```python
from build123d import *

# Parameters (mm, degrees)
EXTRUDE_START            = 27.5
EXTRUDE_1_DEPTH          = 55
SKETCH_4_R               = 10
CUT_EXTRUDE_1_DEPTH      = 55.60082417
CUT_EXTRUDE_2_DEPTH      = 55.60082417
CUT_EXTRUDE_2_DEPTH_BACK = 55.60082417
SKETCH_6_R               = 3.5
CUT_EXTRUDE_3_DEPTH      = 54.937463789
FILLET_1_R               = 2
FILLET_2_R               = 2.8


with BuildPart() as part:
    # 草图3 → 凸台-拉伸1 (new body)
    with BuildSketch(Plane(origin=(0, 0, 0), x_dir=(0, 0, -1), z_dir=(1, 0, 0)).offset(EXTRUDE_START)):
        with BuildLine():
            Line((-28, 0), (-5, 0))
            ThreePointArc((-5, 0), (-1.464466094, 1.464466094), (0, 5))
            Line((0, 5), (0, 40))
            Line((0, 40), (-3, 40))
            Line((-3, 40), (-3, 5))
            ThreePointArc((-3, 5), (-3.585786438, 3.585786438), (-5, 3))
            Line((-5, 3), (-28, 3))
            Line((-28, 3), (-28, 0))
        make_face()
    extrude(amount=-EXTRUDE_1_DEPTH)

    # 草图4 → 切除-拉伸1 (cut, through all)
    with BuildSketch(Plane.XY.offset(3)):
        with Locations((0, 25)):
            Circle(SKETCH_4_R)
    extrude(amount=-CUT_EXTRUDE_1_DEPTH, mode=Mode.SUBTRACT)

    # 草图5 → 切除-拉伸2 (cut, two sides: drawn at the far end of the back side and taken through both)
    with BuildSketch(Plane.XY.offset(3).offset(-CUT_EXTRUDE_2_DEPTH_BACK)):
        Polygon((-17.58587988, 40), (-27.5, 3), (-27.5, 50), (27.5, 50), (27.5, 3), (17.58587988, 40), align=None)
    extrude(amount=CUT_EXTRUDE_2_DEPTH + CUT_EXTRUDE_2_DEPTH_BACK, mode=Mode.SUBTRACT)

    # 草图6 → 切除-拉伸3 (cut, through all)
    with BuildSketch(Plane(origin=(0, 3, 0), x_dir=(1, 0, 0), z_dir=(0, 1, 0))):
        with Locations(Location((-20, -20, 0), (0, 0, 270))):
            Circle(SKETCH_6_R)
        with Locations(Location((20, -20, 0), (0, 0, 90))):
            Circle(SKETCH_6_R)
    extrude(amount=-CUT_EXTRUDE_3_DEPTH, mode=Mode.SUBTRACT)

    # 圆角1
    fillet_1_edges = [part.edges().sort_by_distance(p)[0] for p in [
        (17.58587988, 40, 1.5),
        (-17.58587988, 40, 1.5),
    ]]
    fillet(fillet_1_edges, radius=FILLET_1_R)

    # 圆角2
    fillet_2_edges = [part.edges().sort_by_distance(p)[0] for p in [
        (27.5, 1.5, 28),
        (-27.5, 1.5, 28),
    ]]
    fillet(fillet_2_edges, radius=FILLET_2_R)


solid = part.part
```
The listing builds one solid part. Answer for the finished solid, in the listing's coordinates (mm). A direction names the side the tool comes from. Coordinates: 2 decimals unless noted, no trailing zeros. Loops run counter-clockwise (first coordinate to the right, second up) from the corner with the lowest first, then second, coordinate; pieces in that order, holes last. Notation, with made-up numbers: (34.25, 58) - (53.25, 58) arc R12 cw to (53.25, 80) - close; hole circle Ø11 at (30.5, -18). An arc over 180 degrees is marked (long way). Use a Markdown table: item, result. Add a question column.
1) The part is cut by section B-B, the plane z = 20. Give the vertices of the cut face in (x, y).
2) Find the intervals of material crossed by line 1 (X direction, y = 1.35, z = 20); line 2 (Y direction, x = -11.5, z = 5), in increasing order.
3) The part is cut by section C-C, the plane y = 29. Give the vertices of the cut face in (x, z).
4) The mould has two halves that part along Y. Classify faces 3 (the cylindrical face through (17.05, 1.52, 18.12)), 4 (the cylindrical face through (0.39, 3.6, 3.57)), 5 (the flat face through (0, 0, 17)), 6 (the cylindrical face through (-1.302, 34.915, 1.521)): released by +Y, released by -Y, zero draft, split by the parting line, or undercut.
5) The part is cut by section D-D, the plane x = 13.5. Give the vertices of the cut face in (y, z).
6) Given pin 1 (6.5 mm diameter, centred on x = 20, z = 20, fed in from -Y); pin 2 (6 mm diameter, centred on x = 9, y = 11.5, fed in from +Z); pin 3 (4 mm diameter, centred on x = 1, z = 7, fed in from +Y), each flat-ended and moving along its own axis, determine where each tip first touches the part or whether it passes through.
7) The part is cut by section A-A, the plane x = 1. Give the vertices of the cut face in (y, z), and give its area (3 significant figures).
8) For faces 1 (the flat face through (0, 3, 16)), 2 (the flat face through (27.5, 2, 13)), determine the directions among +Z, -Z, +X, -X, +Y, -Y from which every point of the face is accessible in a straight line to the end or side of a thin tool.
Here are the results:
| question | item | result |
|---|---|---|
| 1 | outline | (-27.5, 0) - (-23.5, 0) - (-23.5, 3) - (-27.5, 3) - close; (-16.5, 0) - (16.5, 0) - (16.5, 3) - (-16.5, 3) - close; (23.5, 0) - (27.5, 0) - (27.5, 3) - (23.5, 3) - close |
| 2 | line 1 | x = -27.5 to -23.5, -16.5 to 16.5, 23.5 to 27.5 |
| 2 | line 2 | y = 0 to 3 |
| 3 | outline | (-20.53, 0) - (-9.17, 0) - (-9.17, 3) - (-20.53, 3) - close; (9.17, 0) - (20.53, 0) - (20.53, 3) - (9.17, 3) - close |
| 4 | face 3 | zero draft |
| 4 | face 4 | released by +Y |
| 4 | face 5 | released by -Y |
| 4 | face 6 | undercut |
| 5 | outline | (0, 5) arc R5 ccw to (5, 0) - (40, 0) - (40, 3) - (5, 3) arc R2 cw to (3, 5) - (3, 28) - (0, 28) - close |
| 6 | pin 1 | passes through |
| 6 | pin 2 | stops at z = 3 |
| 6 | pin 3 | stops at y = 3 |
| 7 | outline | (0, 5) arc R5 ccw to (5, 0) - (15.05, 0) - (15.05, 3) - (5, 3) arc R2 cw to (3, 5) - (3, 28) - (0, 28) - close; (34.95, 0) - (40, 0) - (40, 3) - (34.95, 3) - close |
| 7 | area | 131 mm^2 |
| 8 | face 1 | +Z, +X, -X, +Y |
| 8 | face 2 | +Z, -Z, +X, +Y, -Y |
